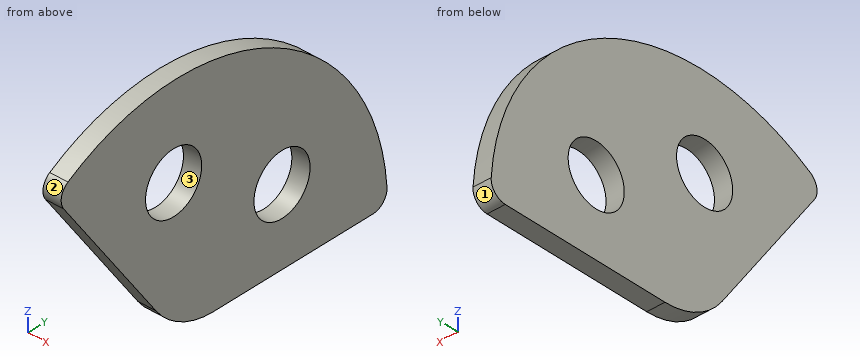
from build123d import *

# Parameters (mm, degrees)
F1_DEPTH = 6
F2_R     = 25
F3_R     = 5
F4_R     = 10
F5_DEPTH = 6.001


with BuildPart() as f1:
    # F0 (on Right) → F1 (new body)
    with BuildSketch(Plane.YZ):
        with BuildLine():
            Line((-43.301281, 61.237236), (0, 0))
            Line((0, 0), (75, 0))
            ThreePointArc((75, 0), (34.477557, 66.605541), (-43.301281, 61.237236))
        make_face()
    extrude(amount=F1_DEPTH)

    # F2
    f2_edges = [f1.edges().sort_by_distance(p)[0] for p in [
        (3, 0, 0),
    ]]
    fillet(f2_edges, radius=F2_R)

    # F3
    f3_edges = [f1.edges().sort_by_distance(p)[0] for p in [
        (3, -43.301281, 61.237236),
        (3, 75, 0),
    ]]
    fillet(f3_edges, radius=F3_R)

    # F4 (on face) → F5 (cut, through all)
    with BuildSketch(Plane.YZ.offset(6)):
        with Locations((-1.190063, 44.984261)):
            Circle(F4_R)
        with Locations((37.416574, 25)):
            Circle(F4_R)
    extrude(amount=-F5_DEPTH, mode=Mode.SUBTRACT)


solid = f1.part
Could you check a few things on this model? Use its own coordinates, in mm. Face numbers are marked on the shaded views. Give positions to 0.01 mm unless a question says otherwise; leave off trailing zeros. Loops run counter-clockwise (first coordinate to the right, second up) from the corner with the lowest first, then second, coordinate; pieces in that order, holes last. Notation, with made-up numbers: (89.25, 77) -> (148.25, 77) arc R15 ccw to (148.25, 97) -> close; hole circle Ø11 at (8, 78.5). An arc over 180 degrees is marked (long way). Return JSON: item names as keys, results as strings.
Item 1: If we section it at A-A on z = 29.5: List the corners of the cut face in (x, y) for me, plus the area to 3 significant figures.
Geometry results:
{"outline": "(0, -20.86) -> (6, -20.86) -> (6, 28.49) -> (0, 28.49) -> close; (0, 46.35) -> (6, 46.35) -> (6, 68.95) -> (0, 68.95) -> close", "area": "432 mm²"}
Item 2: I need wall thicknesses on L1, parallel to Y at x = 3.95, z = 33; L2, parallel to Z at x = 2.3, y = 31; L3, parallel to Y at x = 1.75, z = 24.5. Which ranges of each line are inside material? Lowest first, please. Write a range as from..to.
Geometry results:
{"L1": "y = -23.33..31.42, 43.42..67.35", "L2": "z = 0..17.33, 32.67..68.29", "L3": "y = -17.32..27.43, 47.4..70.89"}
Item 3: I'm going to push flat-ended pins straight in: pin 1 (1 mm diameter, centred on x = 0.5, z = 47, fed in from -Y); pin 2 (2 mm diameter, centred on x = 5, y = 8.5, fed in from -Z); pin 3 (3 mm diameter, centred on x = 5.5, z = 36, fed in from +Y); pin 4 (18 mm diameter, centred on y = -1.19, z = 44.98, fed in from +X) (3 decimals). Where does each tip first touch, or does it pass through?
Geometry results:
{"pin 1": "stops at y = -33.59", "pin 2": "stops at z = 0.24", "pin 3": "stops at y = 66.59", "pin 4": "passes through"}
Item 4: We'd pull the mould along Y, two halves only. Please class the marked faces 1, 2 and 3: +Y half, -Y half, draft (parallel to the pull), parting line (faces both ways), or undercut.
Geometry results:
{"face 1": "+Y half", "face 2": "-Y half", "face 3": "undercut"}
Item 5: If we section it at B-B on y = 44: List the corners of the cut face in (x, z) for me, plus the area to 3 significant figures.
Geometry results:
{"outline": "(0, 0) -> (6, 0) -> (6, 17.47) -> (0, 17.47) -> close; (0, 32.53) -> (6, 32.53) -> (6, 60.74) -> (0, 60.74) -> close", "area": "274 mm²"}
Item 6: If we section it at D-D on y = 59: List the corners of the cut face in (x, z) for me.
Geometry results:
{"outline": "(0, 0) -> (6, 0) -> (6, 46.3) -> (0, 46.3) -> close"}
Item 7: If we section it at C-C on x = 3.5: List the corners of the cut face in (y, z) for me.
Geometry results:
{"outline": "(-40.31, 57.01) -> (-7.47, 10.57) arc R25 ccw to (12.94, 0) -> (69.82, 0) arc R5 ccw to (74.81, 5.36) arc R75 ccw to (-38.82, 64.17) arc R5 ccw to start; hole circle Ø20 at (-1.19, 44.98); hole circle Ø20 at (37.42, 25)"}
